Source: CAD feature listing. Evaluate the final solid. Frame: model axes, mm. Face numbers are marked on the shaded views. Round coordinates to 2 decimals unless told otherwise and drop trailing zeros. Order: outer loops, then holes, each group sorted by start corner. A loop starts at its lowest first (then second) coordinate and runs counter-clockwise, first axis right, second up.
```python
from build123d import *

# Parameters (mm, degrees)
CROQUIS1_W                                           = 195
CROQUIS1_H                                           = 58.7
CROQUIS1_W_2                                         = 153
CROQUIS1_H_2                                         = 31.5
SALIENTE_EXTRUIR1_DEPTH                              = 1.5
REDONDEO1_R                                          = 1
CHAFL_N1_SIZE                                        = 1.4
CORTAR_EXTRUIR1_DEPTH                                = 198.22449138
CROQUIS3_W                                           = 8
CROQUIS3_H                                           = 18
CROQUIS3_H_2                                         = 10
SALIENTE_EXTRUIR2_DEPTH                              = 9
CROQUIS4_W                                           = 174
CROQUIS4_H                                           = 4
CROQUIS4_W_2                                         = 4
CROQUIS4_H_2                                         = 18
CROQUIS4_H_3                                         = 34
SALIENTE_EXTRUIR3_DEPTH                              = 2
REDONDEO2_R                                          = 2
REFRENTADO_PARA_TORNILLO_CON_CABEZA_HUEC_D           = 3.4
REFRENTADO_PARA_TORNILLO_CON_CABEZA_HUEC_CBORE_D     = 6.5
REFRENTADO_PARA_TORNILLO_CON_CABEZA_HUEC_CBORE_DEPTH = 3.4
CHAFL_N2_SIZE                                        = 2
CHAFL_N3_SIZE                                        = 1


with BuildPart() as part:
    # Croquis1 → Saliente-Extruir1 (new body)
    with BuildSketch(Plane.XY):
        with Locations((0, 0.15)):
            Rectangle(CROQUIS1_W, CROQUIS1_H)
        with Locations((0, 0.51)):
            Rectangle(CROQUIS1_W_2, CROQUIS1_H_2, mode=Mode.SUBTRACT)
    extrude(amount=SALIENTE_EXTRUIR1_DEPTH)

    # Redondeo1
    redondeo1_edges = [part.edges().sort_by_distance(p)[0] for p in [
        (-76.5, 16.26, 0.75),
        (-76.5, -15.24, 0.75),
        (76.5, -15.24, 0.75),
        (76.5, 16.26, 0.75),
    ]]
    fillet(redondeo1_edges, radius=REDONDEO1_R)

    # Chaflán1
    chafl_n1_edges = [part.edges().sort_by_distance(p)[0] for p in [
        (-76.5, 0.51, 1.5),
        (0, -15.24, 1.5),
        (76.5, 0.51, 1.5),
        (0, 16.26, 1.5),
        (-76.207106781, -14.947106781, 1.5),
        (76.207106781, -14.947106781, 1.5),
        (76.207106781, 15.967106781, 1.5),
        (-76.207106781, 15.967106781, 1.5),
    ]]
    chamfer(chafl_n1_edges, length=CHAFL_N1_SIZE)

    # Croquis2 → Cortar-Extruir1 (cut, through all)
    with BuildSketch(Plane(origin=(97.5, 0, 0), x_dir=(0, 0, -1), z_dir=(1, 0, 0))):
        Polygon((0, -29.2), (-1.5, -25.078783871), (-1.5, -29.2), align=None)
    extrude(amount=-CORTAR_EXTRUIR1_DEPTH, mode=Mode.SUBTRACT)

    # Croquis3 → Saliente-Extruir2 (add)
    with BuildSketch(Plane(origin=(0, 0, 0), x_dir=(-1, 0, 0), z_dir=(0, 0, -1))):
        with Locations((-91, 18)):
            Rectangle(CROQUIS3_W, CROQUIS3_H)
        with Locations((-91, -18)):
            Rectangle(CROQUIS3_W, CROQUIS3_H)
        with Locations((91, 22)):
            Rectangle(CROQUIS3_W, CROQUIS3_H_2)
        with Locations((91, -22)):
            Rectangle(CROQUIS3_W, CROQUIS3_H_2)
    extrude(amount=SALIENTE_EXTRUIR2_DEPTH)

    # Croquis4 → Saliente-Extruir3 (add)
    with BuildSketch(Plane(origin=(0, 0, 0), x_dir=(-1, 0, 0), z_dir=(0, 0, -1))):
        with Locations((0, 25)):
            Rectangle(CROQUIS4_W, CROQUIS4_H)
        with Locations((0, -25)):
            Rectangle(CROQUIS4_W, CROQUIS4_H)
        with Locations((-93, 0)):
            Rectangle(CROQUIS4_W_2, CROQUIS4_H_2)
        with Locations((93, 0)):
            Rectangle(CROQUIS4_W_2, CROQUIS4_H_3)
    extrude(amount=SALIENTE_EXTRUIR3_DEPTH)

    # Redondeo2
    redondeo2_edges = [part.edges().sort_by_distance(p)[0] for p in [
        (-87, 17, -4.5),
        (-87, -17, -4.5),
        (87, -9, -4.5),
        (87, 9, -4.5),
        (91, -9, -1),
        (87, -23, -1),
        (-87, -23, -1),
        (-91, -17, -1),
        (-91, 17, -1),
        (-87, 23, -1),
        (87, 23, -1),
        (91, 9, -1),
    ]]
    fillet(redondeo2_edges, radius=REDONDEO2_R - 0.0001)  # a hair under: the kernel refuses the full size

    # Refrentado para tornillo con cabeza hueca de M31 (through all)
    with Locations(Plane.XY.offset(1.5)):
        with Locations((-91.5, 23.5), (-91.5, -23.5), (91.5, -23.5), (91.5, 23.5)):
            CounterBoreHole(REFRENTADO_PARA_TORNILLO_CON_CABEZA_HUEC_D / 2, REFRENTADO_PARA_TORNILLO_CON_CABEZA_HUEC_CBORE_D / 2, REFRENTADO_PARA_TORNILLO_CON_CABEZA_HUEC_CBORE_DEPTH)

    # Chaflán2
    chafl_n2_edges = [part.edges().sort_by_distance(p)[0] for p in [
        (-97.5, 29.5, 0.75),
        (97.5, 29.5, 0.75),
    ]]
    chamfer(chafl_n2_edges, length=CHAFL_N2_SIZE)

    # Chaflán3
    chafl_n3_edges = [part.edges().sort_by_distance(p)[0] for p in [
        (0, 29.5, 1.5),
        (-97.5, 1.210608065, 1.5),
        (-96.5, 28.5, 1.5),
        (96.5, 28.5, 1.5),
        (97.5, 1.210608065, 1.5),
    ]]
    chamfer(chafl_n3_edges, length=CHAFL_N3_SIZE)


solid = part.part
```
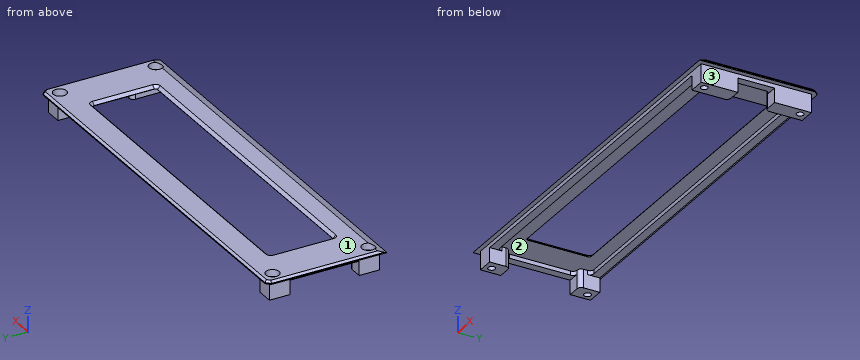
1. First-contact query: pin 1 (6 mm diameter, centred on x = 25.5, y = 16, fed in from -Z); pin 2 (14 mm diameter, centred on x = 16.5, y = -1.5, fed in from -Z); pin 3 (3 mm diameter, centred on x = 30, y = 23, fed in from -Z); pin 4 (1.8 mm diameter, centred on x = 91, z = -3.5, fed in from +Y). Flat tips, straight axial feed; report the tip coordinate or a pass-through.
2. Pull-direction query (X, two-part tool) for the marked faces 1, 2 and 3; classes: released by +X, released by -X, zero draft, split by the parting line, or undercut.
3. Section C-C on y = 1. Return loops of the section in (x, z).
4. Line query: line 1 along Y through (x, z) = (91.5, -0.1); line 2 along X through (y, z) = (-23.5, -1); line 3 along X through (y, z) = (26.5, -6.25). Output: solid intervals per line, ascending.
5. Section B-B on x = 2. Return loops of the section in (y, z).
6. Section A-A on z = -4. Return loops of the section in (x, y), plus the area to 3 significant figures.
Result:
1. pin 1: stops at z = 0
1. pin 2: passes through
1. pin 3: stops at z = -2
1. pin 4: stops at y = 27
2. face 1: zero draft
2. face 2: undercut
2. face 3: released by +X
3. outline: (-97.5, 0) - (-95, 0) - (-95, -2) - (-91, -2) - (-91, 0) - (-76.5, 0) - (-76.5, 0.1) - (-77.9, 1.5) - (-96.5, 1.5) - (-97.5, 0.5) - close; (76.5, 0) - (91, 0) - (91, -2) - (95, -2) - (95, 0) - (97.5, 0) - (97.5, 0.5) - (96.5, 1.5) - (77.9, 1.5) - (76.5, 0.1) - close
4. line 1: y = -27 to -26.75, -20.25 to 20.25, 26.75 to 27
4. line 2: x = -95 to -94.75, -88.25 to 88.25, 94.75 to 95
4. line 3: x = -95 to -87, 87 to 95
5. outline: (-29.2, 0) - (-27, 0) - (-27, -2) - (-23, -2) - (-23, 0) - (-15.24, 0) - (-15.24, 0.1) - (-16.64, 1.5) - (-25.08, 1.5) - close; (16.26, 0) - (23, 0) - (23, -2) - (27, -2) - (27, 0) - (29.5, 0) - (29.5, 0.5) - (28.5, 1.5) - (17.66, 1.5) - (16.26, 0.1) - close
6. outline: (-95, -27) - (-87, -27) - (-87, -19) arc R2 ccw to (-89, -17) - (-95, -17) - close; (-95, 17) - (-89, 17) arc R2 ccw to (-87, 19) - (-87, 27) - (-95, 27) - close; (87, -27) - (95, -27) - (95, -9) - (89, -9) arc R2 ccw to (87, -11) - close; (87, 11) arc R2 ccw to (89, 9) - (95, 9) - (95, 27) - (87, 27) - close; hole circle Ø3.4 at (-91.5, -23.5); hole circle Ø3.4 at (-91.5, 23.5); hole circle Ø3.4 at (91.5, -23.5); hole circle Ø3.4 at (91.5, 23.5)
6. area: 408 mm2
